from build123d import *

# Parameters (mm, degrees)
SKETCH1_W           = 30
SKETCH1_H           = 200
BOSS_EXTRUDE1_DEPTH = 30
SKETCH3_W           = 27.5
SKETCH3_H           = 5
BOSS_EXTRUDE2_DEPTH = 2.6


with BuildPart() as part:
    # Sketch1 → Boss-Extrude1 (new body)
    with BuildSketch(Plane(origin=(0, 0, 0), x_dir=(1, 0, 0), z_dir=(0, 1, 0))):
        Rectangle(SKETCH1_W, SKETCH1_H)
    extrude(amount=BOSS_EXTRUDE1_DEPTH)

    # Sketch3 → Boss-Extrude2 (add)
    with BuildSketch(Plane(origin=(0, 30, 0), x_dir=(1, 0, 0), z_dir=(0, 1, 0))):
        with Locations((0, -87.5)):
            Rectangle(SKETCH3_W, SKETCH3_H)
    boss_extrude2 = extrude(amount=BOSS_EXTRUDE2_DEPTH)

    # Sketch-Pattern1: Boss-Extrude2 at 5 more places
    with Locations((0, 0, -19.5), (0, 0, -79.5), (0, 0, -96.5), (0, 0, -156.5), (0, 0, -173.5)):
        add(boss_extrude2)


solid = part.part
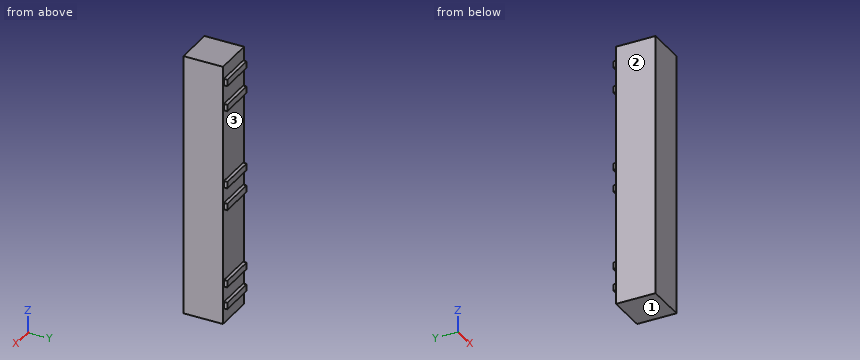
Design review of the part built by this model. Coordinates are the model's own, in mm. Face numbers are marked on the shaded views. Coordinates: 2 decimals unless noted, no trailing zeros. Loops run counter-clockwise (first coordinate to the right, second up) from the corner with the lowest first, then second, coordinate; pieces in that order, holes last. Notation, with made-up numbers: (1, 84.5) - (52, 84.5) arc R17 ccw to (52, 109.5) - close; hole circle Ø7 at (-28, 22.25). An arc over 180 degrees is marked (long way). Use CSV: the item, a comma, the result in double quotes. Start each with the question number.
1. Add section A-A on x = -7. Give the boundary of the cut face in (y, z), plus the area to 3 significant figures.
2. Mouldability with a two-part tool opening along Z and no side actions: class the marked faces 1, 2 and 3 as released by +Z, released by -Z, zero draft, split by the parting line, or undercut.
3. Add section B-B on z = 59.5. Give the boundary of the cut face in (x, y), plus the area to 3 significant figures.
4. Clearance check with flat-ended pins moving along their axes: pin 1 (0.8 mm diameter, centred on y = 31.5, z = -68.5, fed in from +X); pin 2 (5 mm diameter, centred on x = 11.5, z = 47, fed in from -Y); pin 3 (3 mm diameter, centred on x = -3.5, y = 32, fed in from +Z); pin 4 (1.3 mm diameter, centred on x = -2.5, y = 32, fed in from -Z). State where each tip first meets the part, or that it passes through.
5. To check wall thickness, follow probe 1 along Y at (x, z) = (-5.25, -53). State the ranges of the line that lie inside material, in increasing order.
Resolved:
1,outline,"(0, -100) - (30, -100) - (30, -88.5) - (32.6, -88.5) - (32.6, -83.5) - (30, -83.5) - (30, -71.5) - (32.6, -71.5) - (32.6, -66.5) - (30, -66.5) - (30, -11.5) - (32.6, -11.5) - (32.6, -6.5) - (30, -6.5) - (30, 5.5) - (32.6, 5.5) - (32.6, 10.5) - (30, 10.5) - (30, 65.5) - (32.6, 65.5) - (32.6, 70.5) - (30, 70.5) - (30, 85) - (32.6, 85) - (32.6, 90) - (30, 90) - (30, 100) - (0, 100) - close"
1,area,"6,080 mm2"
2,face 1,"released by -Z"
2,face 2,"zero draft"
2,face 3,"undercut"
3,outline,"(-15, 0) - (15, 0) - (15, 30) - (-15, 30) - close"
3,area,"900 mm2"
4,pin 1,"x = 13.75"
4,pin 2,"y = 0"
4,pin 3,"z = 90"
4,pin 4,"z = -88.5"
5,probe 1,"0 to 30"
